```python
from build123d import *

# Parameters (mm, degrees)
SKETCH1_R           = 20
BOSS_EXTRUDE1_DEPTH = 160
BOSS_EXTRUDE2_DEPTH = 110


with BuildPart() as part:
    # Sketch1 → Boss-Extrude1 (new body)
    with BuildSketch(Plane.XY):
        Circle(SKETCH1_R)
    extrude(amount=BOSS_EXTRUDE1_DEPTH)

    # Sketch2 → Boss-Extrude2 (add)
    with BuildSketch(Plane(origin=(0, 0, 0), x_dir=(-1, 0, 0), z_dir=(0, 0, -1))):
        with BuildLine():
            Line((-19.364916731, 5), (-25.478218102, 5))
            Line((-25.478218102, 5), (-25.478218102, -5))
            Line((-25.478218102, -5), (-19.364916731, -5))
            ThreePointArc((-19.364916731, -5), (-20, 0), (-19.364916731, 5))
        make_face()
    extrude(amount=-BOSS_EXTRUDE2_DEPTH)


solid = part.part
```
Here's how the part is built. I have some questions about the finished solid (model axes, mm). A direction names the side the tool comes from. Give positions to 0.01 mm unless a question says otherwise; leave off trailing zeros. Loops run counter-clockwise (first coordinate to the right, second up) from the corner with the lowest first, then second, coordinate; pieces in that order, holes last. Notation, with made-up numbers: M 61,7.5 L 82,7.5 A17 ccw 82,22.5 Z; hole C 58,25.25 d5. An arc over 180 degrees is marked long. Put each result on its own line as item: value. Start each with the question number.
(1) I want a section at B-B on y = 0. Please give me the cut outline in (x, z).
(2) Will these pins go through, and if not, where does the flat tip stop? pin 1 Ø12 at (y, z) = (-13, 56) entering from -X (3 decimals); pin 2 Ø12 at (x, y) = (-4, -15) entering from -Z; pin 3 Ø1.5 at (y, z) = (-10, 35.5) entering from -X; pin 4 Ø10 at (y, z) = (-13, 37) entering from +X.
(3) For faces 1 (the flat face through (22, 5, 54)), 2 (the flat face through (25.478, 0, 54)), 3 (the flat face through (22, -5, 54)), which set-ups out of +Z, -Z, +X, -X, +Y, -Y let a thin tool reach every point of the face, with its end or its side?
(4) I want a section at A-A on z = 147. Please give me the cut outline in (x, y), then the cut area to 3 significant figures.
(5) I want a section at C-C on x = 6.5. Please give me the cut outline in (y, z).
(6) I need wall thicknesses on line 1 along Y through (x, z) = (23, 71); line 2 along X through (y, z) = (1, 60.5); line 3 along X through (y, z) = (3, 148). Which ranges of each line are inside material? Lowest first, please. Write a range as [from, to].
(7) I want a section at D-D on z = 66. Please give me the cut outline in (x, y), then the cut area to 3 significant figures.
Answer block:
1. outline: M -20,0 L 25.48,0 L 25.48,110 L 20,110 L 20,160 L -20,160 Z
2. pin 1: x = -18.735
2. pin 2: z = 0
2. pin 3: x = -17.73
2. pin 4: x = 18.33
3. face 1: +Z, -Z, +X, +Y
3. face 2: +Z, -Z, +X, +Y, -Y
3. face 3: +Z, -Z, +X, -Y
4. outline: C 0,0 d40
4. area: 1,260 mm^2
5. outline: M -18.91,0 L 18.91,0 L 18.91,160 L -18.91,160 Z
6. line 1: [-5, 5]
6. line 2: [-19.97, 25.48]
6. line 3: [-19.77, 19.77]
7. outline: M 19.36,-5 L 25.48,-5 L 25.48,5 L 19.36,5 A20 ccw long Z
7. area: 1,310 mm^2
